```python
from build123d import *

# Parameters (mm, degrees)
ESBO_O1_R                  = 15
ESBO_O1_R_2                = 12.5
RESSALTO_EXTRUS_O1_DEPTH   = 210
RESSALTO_EXTRUS_O3_START   = 15
ESBO_O2_R                  = 12.25
ESBO_O2_R_2                = 10
RESSALTO_EXTRUS_O3_DEPTH   = 20
CORTE_EXTRUS_O2_DEPTH      = 300
CORTE_EXTRUS_O2_DEPTH_BACK = 300
ESBO_O4_R                  = 2.5
ESBO_O9_R                  = 12.5
RESSALTO_EXTRUS_O5_DEPTH   = 10
ESBO_O10_R                 = 10
CORTE_EXTRUS_O5_DEPTH      = 20
ESBO_O7_R                  = 12.5
RESSALTO_EXTRUS_O4_DEPTH   = 10
ESBO_O8_R                  = 10
CORTE_EXTRUS_O4_DEPTH      = 20


with BuildPart() as part:
    # Esbo_o1 → Ressalto-extrus_o1 (new body)
    with BuildSketch(Plane(origin=(0, 0, 0), x_dir=(0, 0, -1), z_dir=(1, 0, 0))):
        Circle(ESBO_O1_R)
        Circle(ESBO_O1_R_2, mode=Mode.SUBTRACT)
    extrude(amount=RESSALTO_EXTRUS_O1_DEPTH)

    # Esbo_o4 → Corte-extrus_o2 (cut, two sides: drawn at the far end of the back side and taken through both)
    with BuildSketch(Plane(origin=(0, 0, 0), x_dir=(1, 0, 0), z_dir=(0, 1, 0)).offset(-CORTE_EXTRUS_O2_DEPTH_BACK)):
        with Locations(Location((205, 0, 0), (0, 0, 90))):
            Circle(ESBO_O4_R)
    extrude(amount=CORTE_EXTRUS_O2_DEPTH + CORTE_EXTRUS_O2_DEPTH_BACK, mode=Mode.SUBTRACT)



with BuildPart() as body_2:
    # Esbo_o2 → Ressalto-extrus_o3 (new body)
    with BuildSketch(Plane.ZY.offset(RESSALTO_EXTRUS_O3_START)):
        Circle(ESBO_O2_R)
        Circle(ESBO_O2_R_2, mode=Mode.SUBTRACT)
    extrude(amount=-RESSALTO_EXTRUS_O3_DEPTH)


with BuildPart() as part_1:
    add(part.part)

    add(body_2.part)  # Ressalto-extrus_o5 merges body 2
    # Esbo_o9 → Ressalto-extrus_o5 (add)
    with BuildSketch(Plane.ZY):
        Circle(ESBO_O9_R)
    extrude(amount=-RESSALTO_EXTRUS_O5_DEPTH)

    # Esbo_o10 → Corte-extrus_o5 (cut)
    with BuildSketch(Plane.ZY):
        Circle(ESBO_O10_R)
    extrude(amount=-CORTE_EXTRUS_O5_DEPTH, mode=Mode.SUBTRACT)

    # Esbo_o7 → Ressalto-extrus_o4 (add)
    with BuildSketch(Plane.ZY):
        Circle(ESBO_O7_R)
    extrude(amount=-RESSALTO_EXTRUS_O4_DEPTH)

    # Esbo_o8 → Corte-extrus_o4 (cut)
    with BuildSketch(Plane.ZY):
        Circle(ESBO_O8_R)
    extrude(amount=-CORTE_EXTRUS_O4_DEPTH, mode=Mode.SUBTRACT)


solid = part_1.part
```
Design review of the part built by this model. Coordinates are the model's own, in mm. A direction names the side the tool comes from. Coordinates: 2 decimals unless noted, no trailing zeros. Loops run counter-clockwise (first coordinate to the right, second up) from the corner with the lowest first, then second, coordinate; pieces in that order, holes last. Notation, with made-up numbers: (-24, 65.25) - (-1, 65.25) arc R34 cw to (-1, 96.25) - close; hole circle Ø10 at (-35.75, 30). An arc over 180 degrees is marked (long way). Use CSV: the item, a comma, the result in double quotes. Start each with the question number.
1) Consider section B-B on y = 0. Write out the cut boundary in (x, z).
2) Tool access review of faces 1 (the cylindrical face through (108.6, 3.755, -11.923)), 2 (the cylindrical face through (-2.68, -9.76, -2.17)), 3 (the cylindrical face through (-7.605, 10.329, 6.586)): name each direction out of +Z, -Z, +X, -X, +Y, -Y from which nothing blocks a thin tool from reaching the whole face with its end or side.
3) For pin 1 Ø10 at (x, z) = (162, -10) entering from +Y; pin 2 Ø8 at (y, z) = (8.5, -4.5) entering from +X; pin 3 Ø4 at (x, y) = (122, -8) entering from +Z; pin 4 Ø6 at (x, z) = (44.5, 9.5) entering from +Y, all flat-tipped, find the tip position at first contact; note any pin that passes through.
4) Consider section C-C on x = 205. Write out the cut boundary in (y, z), then the cut area to 3 significant figures.
5) The part is to be moulded in two halves that separate along X. For faces 4 (the cylindrical face through (203.31, -13.64, 1.84)), 5 (the flat face through (210, 12.3, 3.4)), 6 (the flat face through (-15, -9, -5)), 7 (the cylindrical face through (204.9, 13.6, 2.5)), say which applies: +X half, -X half, draft (parallel to the pull), parting line (faces both ways), or undercut.
6) Consider section A-A on z = 0. Write out the cut boundary in (x, y), then the cut area to 3 significant figures.
7) Wall thickness on L1, parallel to Y at x = -6.5, z = 0; L2, parallel to Y at x = 4.75, z = 0; L3, parallel to Z at x = 29, y = -1: over which ranges is each line inside the solid? List them lowest first. Write a range as from..to.
Geometry says:
1,outline,"(-15, -12.25) - (0, -12.25) - (0, -15) - (210, -15) - (210, -12.5) - (10, -12.5) - (10, -10) - (-15, -10) - close; (-15, 10) - (10, 10) - (10, 12.5) - (210, 12.5) - (210, 15) - (0, 15) - (0, 12.25) - (-15, 12.25) - close"
2,face 1,"+X"
2,face 2,"+X, -X"
2,face 3,"-X"
3,pin 1,"y = 14.14"
3,pin 2,"x = 210"
3,pin 3,"z = 13.75"
3,pin 4,"y = 13.52"
4,outline,"(-14.79, -2.5) arc R15 ccw to (14.79, -2.5) - (12.25, -2.5) arc R12.5 cw to (-12.25, -2.5) - close; (-14.79, 2.5) - (-12.25, 2.5) arc R12.5 cw to (12.25, 2.5) - (14.79, 2.5) arc R15 ccw to start"
4,area,"191 mm^2"
5,face 4,"undercut"
5,face 5,"+X half"
5,face 6,"-X half"
5,face 7,"undercut"
6,outline,"(-15, -12.25) - (0, -12.25) - (0, -15) - (202.5, -15) - (202.5, -12.5) - (10, -12.5) - (10, -10) - (-15, -10) - close; (-15, 10) - (10, 10) - (10, 12.5) - (202.5, 12.5) - (202.5, 15) - (0, 15) - (0, 12.25) - (-15, 12.25) - close; (207.5, -15) - (210, -15) - (210, -12.5) - (207.5, -12.5) - close; (207.5, 12.5) - (210, 12.5) - (210, 15) - (207.5, 15) - close"
6,area,"1,140 mm^2"
7,L1,"-12.25..-10, 10..12.25"
7,L2,"-15..-10, 10..15"
7,L3,"-14.97..-12.46, 12.46..14.97"
